The model under review builds one solid part; all positions refer to its coordinate system, in mm. A direction names the side the tool comes from. Round coordinates to 2 decimals unless told otherwise and drop trailing zeros. Write each loop counter-clockwise with the first axis right and the second up, starting at its lowest first coordinate (ties: lowest second). Pieces come first, ordered by that corner, then holes. Notation, with made-up numbers: (50, 86.5) - (58, 86.5) arc R30 ccw to (58, 124.5) - close; hole circle Ø2 at (28.25, 83.25). An arc over 180 degrees is marked (long way). Return JSON: item names as keys, results as strings.
Autodesk Fusion 360 part; units mm, degrees
sketch "Sketch1" plane through (0, 0, 0) normal (0, 0, 1) x (1, 0, 0)
  line L0 (-1.9341, 3.35) -> (-3.8682, 0)
  line L1 (-3.8682, 0) -> (-1.9341, -3.35)
  line L2 (-1.9341, -3.35) -> (1.9341, -3.35)
  line L3 (1.9341, -3.35) -> (3.8682, 0)
  line L4 (3.8682, 0) -> (1.9341, 3.35)
  line L5 (1.9341, 3.35) -> (-1.9341, 3.35)
  line L6 (-0.6, 5.5) -> (-0.6, -5.5)
  line L7 (0, 2.5) -> (0, 20) construction
  line L8 (0.6, 5.5) -> (0.6, -5.5)
  line L9 (-6.3509, 0) -> (-3.1754, -5.5)
  line L10 (-3.1754, -5.5) -> (3.1754, -5.5)
  line L11 (3.1754, -5.5) -> (6.3509, 0)
  line L12 (6.3509, 0) -> (3.1754, 5.5)
  line L13 (3.1754, 5.5) -> (-3.1754, 5.5)
  line L14 (-3.1754, 5.5) -> (-6.3509, 0)
  dimension "d1" = 6.7
  dimension "d3" = 1.2
  dimension "d14" = 11
extrude "Extrude1" add sketch "Sketch1" along normal blind 13 contours L0 L1 L2 L5 L6 L9 L10 L13 L14 | L5 L6 L8 L13 | L2 L3 L4 L5 L8 L10 L11 L12 L13 | L2 L6 L8 L10
extrude "Extrude2" add sketch "Sketch1" along normal blind 6 from surface at 13
extrude "Extrude3" add sketch "Sketch1" along normal blind 8 from surface at 19 contours L0 L1 L2 L5 L6 | L0 L1 L2 L5 L6 L9 L10 L13 L14 | L2 L3 L4 L5 L8 L10 L11 L12 L13 | L2 L3 L4 L5 L8
chamfer "Chamfer1" distance 1 angle 45 2 edges at (0.6, 0, 27) (-0.6, 0, 27)
sketch "Sketch2" plane through (0, 0, 0) normal (0, 1, 0) x (1, 0, 0)
  line L0 (3.8682, -13) -> (-3.8682, -13)
  line L1 (-3.8682, -13) -> (-3.8682, 0)
  line L2 (-3.8682, 0) -> (-6.3509, 0)
  line L3 (-6.3509, 0) -> (-6.3509, -27)
  line L4 (-6.3509, -27) -> (-1.6, -27)
  line L5 (-1.6, -27) -> (-0.6, -26)
  line L6 (-0.6, -26) -> (-0.6, -19)
  line L7 (-0.6, -19) -> (0.6, -19)
  line L8 (0.6, -19) -> (0.6, -26)
  line L9 (0.6, -26) -> (1.6, -27)
  line L10 (1.6, -27) -> (6.3509, -27)
  line L11 (6.3509, -27) -> (6.3509, 0)
  line L12 (6.3509, 0) -> (3.8682, 0)
  line L13 (3.8682, 0) -> (3.8682, -13)
  line L14 (-1.6, -27) -> (1.6, -27) construction
  line L15 (0, -27) -> (0, -26.8393) construction
  arc A0 (2.6, -27) -> (6.3509, -23.2491) centre (2.6, -23.2491) ccw
  line L16 (3.1754, -27) -> (1.6, -27)
  dimension "d15" = 1
revolve "Revolve1" cut sketch "Sketch2" angle 360 about axis through (0, 0, 1.75) along (0, 0, 1) contours L10 L11 A0 L16
(1) Add section B-B (z = 22.5). Write out the cut boundary in (x, y), plus the area to 3 significant figures.
Filled in:
{"outline": "(-6.35, 0) - (-3.18, -5.5) - (-0.6, -5.5) - (-0.6, 5.5) - (-3.18, 5.5) - close; (0.6, -5.5) - (3.18, -5.5) - (6.35, 0) - (3.18, 5.5) - (0.6, 5.5) - close", "area": "91.6 mm2"}
(2) Add section A-A (z = 7). Write out the cut boundary in (x, y), plus the area to 3 significant figures.
Filled in:
{"outline": "(-6.35, 0) - (-3.18, -5.5) - (3.18, -5.5) - (6.35, 0) - (3.18, 5.5) - (-3.18, 5.5) - close; hole (-3.87, 0) - (-1.93, -3.35) - (1.93, -3.35) - (3.87, 0) - (1.93, 3.35) - (-1.93, 3.35) - close", "area": "65.9 mm2"}
(3) Clearance check with flat-ended pins moving along their axes: pin 1 Ø3 at (y, z) = (-4, 8) entering from -X; pin 2 Ø1.3 at (x, y) = (0, -2.5) entering from +Z; pin 3 Ø3.5 at (x, y) = (-2, -1) entering from -Z; pin 4 Ø1.5 at (x, y) = (1, -4) entering from +Z. State where each tip first meets the part, or that it passes through.
Filled in:
{"pin 1": "stops at x = -4.91", "pin 2": "stops at z = 26.05", "pin 3": "stops at z = 0", "pin 4": "stops at z = 26.84"}
(4) For faces 1 (the flat face through (1.1, -0.1, 26.5)), 2 (the flat face through (-2, 0, 27)), 3 (the flat face through (-2.888, 1.698, 6.409)), list the 3-axis set-ups (+Z, -Z, +X, -X, +Y, -Y) from which the entire face can be reached by the end or side of a thin tool; tool diameter is ignored.
Filled in:
{"face 1": "+Z, +Y, -Y", "face 2": "+Z, +X, -X, +Y, -Y", "face 3": "-Z"}
(5) Mouldability with a two-part tool opening along X and no side actions: class faces 4 (the flat face through (0, 0, 13)), 5 (the flat face through (0, 5.5, 13)), 6 (the flat face through (-4.74, 2.79, 12.63)) as released by +X, released by -X, zero draft, split by the parting line, or undercut.
Filled in:
{"face 4": "undercut", "face 5": "zero draft", "face 6": "released by -X"}
(6) Wall thickness on line 1 (Y direction, x = 1.5, z = 12.5); line 2 (X direction, y = 2, z = 8.25); line 3 (X direction, y = -3, z = 25.25): over which ranges is each line inside the solid? List them lowest first.
Filled in:
{"line 1": "y = -5.5 to -3.35, 3.35 to 5.5", "line 2": "x = -5.2 to -2.71, 2.71 to 5.2", "line 3": "x = -4.62 to -0.6, 0.6 to 4.62"}
(7) Add section C-C (z = 15.5). Write out the cut boundary in (x, y).
Filled in:
{"outline": "(-6.35, 0) - (-3.18, -5.5) - (3.18, -5.5) - (6.35, 0) - (3.18, 5.5) - (-3.18, 5.5) - close"}
